```python
from build123d import *

# Parameters (mm, degrees)
SKETCH1_R          = 20.5
SKETCH1_R_2        = 12.5
SKETCH1_R_3        = 1.5875
EXTRUDE1_DEPTH     = 5
CUT_EXTRUDE1_DEPTH = 30.419381367
CIRPATTERN1_COUNT  = 3
SKETCH3_W          = 2.5
SKETCH3_H          = 2.5
SKETCH4_W          = 20.5
SKETCH4_H          = 1.5
CUT_EXTRUDE2_DEPTH = 30.201883501


with BuildPart() as part:
    # Sketch1 → Extrude1 (new body)
    with BuildSketch(Plane.XY):
        Circle(SKETCH1_R)
        Circle(SKETCH1_R_2, mode=Mode.SUBTRACT)
        with Locations((0, 16.5)):
            Circle(SKETCH1_R_3, mode=Mode.SUBTRACT)
        with Locations((14.289419162, -8.25)):
            Circle(SKETCH1_R_3, mode=Mode.SUBTRACT)
        with Locations((-14.289419162, -8.25)):
            Circle(SKETCH1_R_3, mode=Mode.SUBTRACT)
    extrude(amount=EXTRUDE1_DEPTH)

    # Sketch2 → Cut-Extrude1 (cut, through all)
    with BuildSketch(Plane.XY.offset(5)):
        with BuildLine():
            ThreePointArc((1.5, -16.5), (0, -15), (-1.5, -16.5))
            Line((-1.5, -16.5), (-1.5, -20.4450483))
            ThreePointArc((-1.5, -20.4450483), (0, -20.5), (1.5, -20.4450483))
            Line((1.5, -20.4450483), (1.5, -16.5))
        make_face()
    cut_extrude1 = extrude(amount=-CUT_EXTRUDE1_DEPTH, mode=Mode.SUBTRACT)

    # CirPattern1: Cut-Extrude1 ×3 about axis
    cirpattern1_axis = Axis((0, 0, 0), (0, 0, 1))
    for i in range(1, CIRPATTERN1_COUNT):
        add(cut_extrude1.rotate(cirpattern1_axis, i * 360 / CIRPATTERN1_COUNT), mode=Mode.SUBTRACT)

    # Sketch3 → Revolve1 (revolve)
    with BuildSketch(Plane(origin=(0, 0, 0), x_dir=(1, 0, 0), z_dir=(0, 1, 0))):
        with Locations((-11.25, -3.75)):
            Rectangle(SKETCH3_W, SKETCH3_H)
    revolve(axis=Axis((0, 0, 0), (0, 0, 1)))

    # Sketch4 → Cut-Revolve1 (revolve, cut)
    with BuildSketch(Plane(origin=(0, 0, 0), x_dir=(1, 0, 0), z_dir=(0, 1, 0))):
        with Locations((-10.25, -0.75)):
            Rectangle(SKETCH4_W, SKETCH4_H)
    revolve(axis=Axis((0, 0, 0), (0, 0, 1)), mode=Mode.SUBTRACT)

    # Sketch5 → Cut-Extrude2 (cut, through all)
    with BuildSketch(Plane.XY.offset(5)):
        with BuildLine():
            ThreePointArc((-1.5, -16.5), (-1.060660172, -15.439339828), (0, -15))
            Line((0, -15), (-3, -15))
            ThreePointArc((-3, -15), (-4.060660172, -15.439339828), (-4.5, -16.5))
            Line((-4.5, -16.5), (-4.5, -20))
            ThreePointArc((-4.5, -20), (-3.008241512, -20.278078878), (-1.5, -20.4450483))
            Line((-1.5, -20.4450483), (-1.5, -16.5))
        make_face()
    extrude(amount=-CUT_EXTRUDE2_DEPTH, mode=Mode.SUBTRACT)

    # Sketch6 → Cut-Revolve2 (revolve, cut)
    with BuildSketch(Plane(origin=(0, 0, 0), x_dir=(1, 0, 0), z_dir=(0, 1, 0))):
        Polygon((-10, -5), (-12.045348365, -2.5), (-10, -2.5), align=None)
    revolve(axis=Axis((0, 0, 0), (0, 0, 1)), mode=Mode.SUBTRACT)


solid = part.part
```
Geometry: final body of the model. Coordinates: model frame, mm. A direction names the side the tool comes from. Coordinates: 2 decimals unless noted, no trailing zeros. Write each loop counter-clockwise with the first axis right and the second up, starting at its lowest first coordinate (ties: lowest second). Pieces come first, ordered by that corner, then holes. Notation, with made-up numbers: M 71.5,82.25 L 92.5,82.25 A31 ccw 92.5,115.25 Z; hole C 31,44.25 d11. An arc over 180 degrees is marked long. Use CSV: the item, a comma, the result in double quotes. Start each with the question number.
1. Cut plane A-A on y = 0. Return the cut outline in (x, z).
2. Mould query, pull axis X, two halves, no side actions, for faces 4 (the face through (9, 9, 1.5)), 5 (the face through (1.5, -19, 3)), 6 (the face through (-15.22, 10.52, 3.27)). Classes: pulls with the +X half, pulls with the -X half, needs draft (parallel to the pull), parting line crosses it, or undercut.
3. Cut plane C-C on y = 16.5. Return the cut outline in (x, z).
4. Ray query, probe 1 along X at (y, z) = (0.5, 2.1); probe 2 along X at (y, z) = (-8.25, 2.45); probe 3 along X at (y, z) = (-9.5, 1.8). Return the intervals inside material, ascending.
5. Cut plane B-B on z = 2. Count the separate pieces of the cut face and the enclosed holes in it, plus the area to 3 significant figures.
6. Cut plane D-D on x = -17.5. Return the cut outline in (y, z), plus the area to 3 significant figures.
7. Reachability of faces 1 (the face through (-4.5, -18, 3)), 2 (the face through (-16.77, 7.95, 3.27)), 3 (the face through (11.923, 3.755, 1.993)) from +Z, -Z, +X, -X, +Y, -Y: full face, straight path, thin tool, end or side. Return the list, or none.
8. First-contact query: P1, Ø1, axis at y = -18, z = 2.5, coming from the -X side; P2, Ø1.5, axis at y = 12.5, z = 4.5, coming from the -X side; P3, Ø2.5, axis at x = 0, y = 16.5, coming from the -Z side; P4, Ø0.9, axis at x = -1.5, z = 2.5, coming from the -Y side. Flat tips, straight axial feed; report the tip coordinate or a pass-through.
Entries:
1,outline,"M -20.5,1.5 L -12.5,1.5 L -12.5,2.5 L -12.05,2.5 L -10,5 L -20.5,5 Z; M 10,5 L 12.05,2.5 L 12.5,2.5 L 12.5,1.5 L 20.5,1.5 L 20.5,5 Z"
2,face 4,"needs draft"
2,face 5,"undercut"
2,face 6,"pulls with the -X half"
3,outline,"M -12.17,1.5 L -1.59,1.5 L -1.59,5 L -12.17,5 Z; M 1.59,1.5 L 12.17,1.5 L 12.17,5 L 1.59,5 Z"
4,probe 1,"-20.49 to -12.49, 12.49 to 20.49"
4,probe 2,"-18.77 to -15.88, -12.7 to -9.39, 9.39 to 12.7, 15.88 to 18.77"
4,probe 3,"-18.17 to -15.27, -13.31 to -8.12, 8.12 to 13.31, 15.27 to 18.17"
5,separate pieces,"1"
5,enclosed holes,"4"
5,area,"743 mm²"
6,outline,"M -10.68,1.5 L 8.37,1.5 L 8.37,5 L -10.68,5 Z"
6,area,"66.7 mm²"
7,face 1,"+Z, -Z, -Y"
7,face 2,"+Z, -Z"
7,face 3,"-Z"
8,P1,"x = -10.68"
8,P2,"x = -16.8"
8,P3,"through"
8,P4,"y = -15"
